from build123d import *

# Parameters (mm, degrees)
SKETCH_1_W           = 195.008255005
SKETCH_1_H           = 479.009395123
EXTRUDE_2_DEPTH      = 135
CUT_EXTRUDE_4_DEPTH  = 200
CUT_EXTRUDE_23_DEPTH = 200


with BuildPart() as part:
    # Эскиз1 → Бобышка-Вытянуть2 (new body)
    with BuildSketch(Plane(origin=(0, 0, 0), x_dir=(1, 0, 0), z_dir=(0, 1, 0))):
        with Locations((97.504127503, 243.967165232)):
            Rectangle(SKETCH_1_W, SKETCH_1_H)
    extrude(amount=EXTRUDE_2_DEPTH)

    # Эскиз3 → Вырез-Вытянуть4 (cut)
    with BuildSketch(Plane.ZY):
        Polygon((-483.471862793, 40.937199902), (-245.760530455, 135), (-483.471862793, 135), align=None)
        Polygon((-108.474701812, 135), (-243.967165232, 135), (-190.717834923, 59.88686474), (-108.474701812, 59.88686474), align=None)
        Polygon((-4.46246767, 135), (-96.73151757, 135), (-93.463282811, 59.88686474), (-60.345170592, 59.88686474), (-53.808701075, 116.435636272), (-4.46246767, 116.435636272), align=None)
        Polygon((-4.46246767, 10.364015235), (-483.471862793, 3.305962882), (-483.471862793, 0), (-4.46246767, 0), align=None)
    extrude(amount=-CUT_EXTRUDE_4_DEPTH, mode=Mode.SUBTRACT)

    # Эскиз4 → Вырез-Вытянуть23 (cut)
    with BuildSketch(Plane(origin=(0, 200.805738218, -79.459190383), x_dir=(1, 0, 0), z_dir=(0, 0.9298484645549542, -0.3679427033721343))):
        Polygon((53.747628165, 434.493025273), (140.455159465, 434.493025273), (143.17020938, 491.267849843), (50.129149916, 491.267849843), align=None)
        Polygon((132.896060194, 276.42354275), (140.455159465, 434.493025273), (53.747628165, 434.493025273), (63.82200512, 276.42354275), align=None)
        Polygon((0, 434.493025273), (19.603729829, 434.493025273), (27.465109106, 491.267849843), (0, 491.267849843), align=None)
        Polygon((0, 434.493025273), (0, 292.915029518), (19.603729829, 434.493025273), align=None)
        Polygon((174.530095187, 434.493025273), (195.008255005, 285.726840395), (195.008255005, 434.493025273), align=None)
        Polygon((174.477407826, 434.875779277), (174.530095187, 434.493025273), (195.008255005, 434.493025273), (195.008255005, 491.267849843), (166.714851877, 491.267849843), align=None)
    extrude(amount=-CUT_EXTRUDE_23_DEPTH, mode=Mode.SUBTRACT)


solid = part.part
Here's how the part is built. I have some questions about the finished solid (model axes, mm). A direction names the side the tool comes from. Coordinates: 2 decimals unless noted, no trailing zeros. Order: outer loops, then holes, each group sorted by start corner. A loop starts at its lowest first (then second) coordinate and runs counter-clockwise, first axis right, second up. Notation, with made-up numbers: M 17.5,38.5 L 75.5,38.5 A19 ccw 75.5,65.5 Z; hole C 27.25,3.5 d1. An arc over 180 degrees is marked long. Answer as CSV lines item,"result". Start each with the question number.
1. On a 3-axis mill with a long thin cutter (end or side, diameter ignored), from which of +Z, -Z, +X, -X, +Y, -Y can I reach the whole of each face in a straight line? I mean faces 4 (the flat face through (96, 116.436, -29)), 5 (the flat face through (96, 59.887, -150)), 6 (the flat face through (96, 63, -4.462)). Say none if no direction works.
2. I want a section at C-C, the plane z = -325. Write out the boundary of the cut face in (x, y).
3. I want a section at B-B, the plane x = 37. Write out the boundary of the cut face in (y, z).
4. I want a section at A-A, the plane y = 68.5. Write out the boundary of the cut face in (x, z).
5. I need wall thicknesses on line 1 (Z direction, x = 124, y = 99); line 2 (Z direction, x = 103, y = 85); line 3 (X direction, y = 67, z = -354.5). Which ranges of each line are inside material? Lowest first, please. Write a range as [from, to].
6. For pin 1 (10 mm diameter, centred on x = 90.5, z = -69, fed in from +Y); pin 2 (6 mm diameter, centred on x = 153.5, z = -115, fed in from -Y); pin 3 (1 mm diameter, centred on x = 130.5, z = -253.5, fed in from -Y), each with a flat end and sliding along its axis, tell me the tip position at first contact or that it passes through.
7. I want a section at D-D, the plane y = 25. Write out the boundary of the cut face in (x, z).
8. We'd pull the mould along X, two halves only. Please class faces 1 (the flat face through (0, 55, -176)), 2 (the flat face through (96.14, 108.21, -313.46)), 3 (the flat face through (97.876, 53.208, -318.332)): released by +X, released by -X, zero draft, split by the parting line, or undercut.
Recorded:
1,face 4,"+Z, +X, -X, +Y"
1,face 5,"+X, -X, +Y"
1,face 6,"+Z, +X, -X, +Y, -Y"
2,outline,"M 0,25.24 L 1,5.64 L 62.31,5.64 L 63.82,70.06 L 132.9,70.06 L 134.03,5.64 L 193.03,5.64 L 195.01,44.77 L 195.01,103.64 L 0,103.64 Z"
3,outline,"M 3.31,-483.47 L 40.94,-483.47 L 135,-245.76 L 135,-243.97 L 59.89,-190.72 L 59.89,-108.47 L 135,-108.47 L 135,-96.73 L 59.89,-93.46 L 59.89,-60.35 L 116.44,-53.81 L 116.44,-4.46 L 10.36,-4.46 Z"
4,outline,"M 0,-342.12 L 9.23,-413.82 L 58.52,-413.82 L 63.82,-324.38 L 132.9,-324.38 L 136.87,-413.82 L 184.84,-413.82 L 195.01,-334.39 L 195.01,-196.82 L 0,-196.82 Z; M 0,-108.47 L 195.01,-108.47 L 195.01,-93.84 L 0,-93.84 Z; M 0,-59.35 L 195.01,-59.35 L 195.01,-4.46 L 0,-4.46 Z"
5,line 1,"z = [-336.45, -218.45], [-108.47, -95.17], [-55.82, -4.46]"
5,line 2,"z = [-330.91, -208.52], [-108.47, -94.56], [-57.44, -4.46]"
5,line 3,"x = [1.67, 62], [134.26, 192.36]"
6,pin 1,"stops at y = 59.89"
6,pin 2,"stops at y = 8.69"
6,pin 3,"stops at y = 6.69"
7,outline,"M 0,-324.91 L 20.42,-483.47 L 53.37,-483.47 L 63.82,-307.17 L 132.9,-307.17 L 140.74,-483.47 L 173.72,-483.47 L 195.01,-317.18 L 195.01,-4.46 L 0,-4.46 Z"
8,face 1,"released by -X"
8,face 2,"zero draft"
8,face 3,"undercut"
